```python
from build123d import *

# Parameters (mm, degrees)
SKETCH2_R               = 14.3129
SKETCH2_R_2             = 3.175
SKETCH2_R_3             = 2.6035
SKETCH2_R_4             = 3.2639
BOSS_EXTRUDE1_DEPTH     = 9.525
CHAMFER1_SIZE           = 4.7625
SKETCH3_R               = 2.6035
CUT_EXTRUDE1_DEPTH      = 25.4
CUT_EXTRUDE2_REACH      = 290.278
CUT_EXTRUDE2_END_RADIUS = 14.3129
SKETCH4_R               = 2.6035


with BuildPart() as part:
    # Sketch2 → Boss-Extrude1 (new body)
    with BuildSketch(Plane(origin=(-47.625, 0, 0), x_dir=(0, 0, -1), z_dir=(1, 0, 0))):
        with BuildLine():
            Line((51.301650802, 73.15), (51.301650802, 85.85))
            Line((51.301650802, 85.85), (24.65662816, 193.550056376))
            ThreePointArc((24.65662816, 193.550056376), (0, 212.85), (-24.65662816, 193.550056376))
            Line((-24.65662816, 193.550056376), (-51.301650802, 85.85))
            Line((-51.301650802, 85.85), (-51.301650802, 73.15))
            Line((-51.301650802, 73.15), (-51.301650802, -66.8))
            Line((-51.301650802, -66.8), (51.301650802, -66.8))
            Line((51.301650802, -66.8), (51.301650802, 73.15))
        make_face()
        with Locations(Location((0, 187.45, 0), (0, 0, 180))):
            Circle(SKETCH2_R, mode=Mode.SUBTRACT)
        with Locations(Location((38.476238101, 74.7375, 0), (0, 0, 180))):
            Circle(SKETCH2_R_2, mode=Mode.SUBTRACT)
        with Locations(Location((0, 74.7375, 0), (0, 0, 180))):
            Circle(SKETCH2_R_2, mode=Mode.SUBTRACT)
        with Locations(Location((-38.476238101, 74.7375, 0), (0, 0, 180))):
            Circle(SKETCH2_R_2, mode=Mode.SUBTRACT)
        with Locations(Location((0, 136.65, 0), (0, 0, 180))):
            Circle(SKETCH2_R_3, mode=Mode.SUBTRACT)
        with Locations(Location((-25.4, 136.65, 0), (0, 0, 180))):
            Circle(SKETCH2_R_3, mode=Mode.SUBTRACT)
        with Locations(Location((-31.75, 104.9, 0), (0, 0, 180))):
            Circle(SKETCH2_R_3, mode=Mode.SUBTRACT)
        with Locations(Location((0, 104.9, 0), (0, 0, 180))):
            Circle(SKETCH2_R_3, mode=Mode.SUBTRACT)
        with Locations(Location((31.75, 104.9, 0), (0, 0, 180))):
            Circle(SKETCH2_R_3, mode=Mode.SUBTRACT)
        with Locations(Location((25.4, 136.65, 0), (0, 0, 180))):
            Circle(SKETCH2_R_3, mode=Mode.SUBTRACT)
        with Locations(Location((-25.4, 155.7, 0), (0, 0, 180))):
            Circle(SKETCH2_R_4, mode=Mode.SUBTRACT)
        with Locations(Location((25.4, 155.7, 0), (0, 0, 180))):
            Circle(SKETCH2_R_4, mode=Mode.SUBTRACT)
    extrude(amount=BOSS_EXTRUDE1_DEPTH)

    # Chamfer1
    chamfer1_edges = [part.edges().sort_by_distance(p)[0] for p in [
        (-47.625, 74.7375, -3.175),
        (-47.625, 74.7375, -41.651238101),
        (-47.625, 74.7375, 35.301238101),
    ]]
    chamfer(chamfer1_edges, length=CHAMFER1_SIZE)

    # Sketch3 → Cut-Extrude1 (cut)
    with BuildSketch(Plane.XZ.offset(66.8)):
        with Locations(Location((-42.8625, -38.476238101, 0), (0, 0, 270))):
            Circle(SKETCH3_R)
        with Locations(Location((-42.8625, 0, 0), (0, 0, 270))):
            Circle(SKETCH3_R)
        with Locations(Location((-42.8625, 38.476238101, 0), (0, 0, 90))):
            Circle(SKETCH3_R)
    extrude(amount=-CUT_EXTRUDE1_DEPTH, mode=Mode.SUBTRACT)

    # Cut-Extrude2: up to this cylinder (the profile starts outside it)
    cut_extrude2_end = Plane(origin=(-42.8625, 187.45, 0), z_dir=(-1, 0, 0)) * Cylinder(CUT_EXTRUDE2_END_RADIUS, 610.1818, mode=Mode.PRIVATE)
    # Sketch4 → Cut-Extrude2 (cut, up to the surface)
    with BuildSketch(Plane(origin=(0, 212.85, 0), x_dir=(-1, 0, 0), z_dir=(0, 1, 0)), mode=Mode.PRIVATE) as cut_extrude2_sk1:
        with Locations(Location((42.8625, 0, 0), (0, 0, 270))):
            Circle(SKETCH4_R)
    cut_extrude2_tool1 = extrude(cut_extrude2_sk1.sketch, amount=-CUT_EXTRUDE2_REACH, mode=Mode.PRIVATE) - cut_extrude2_end
    add(cut_extrude2_tool1.solids().sort_by_distance((-42.8625, 212.85, 0))[0], mode=Mode.SUBTRACT)


solid = part.part
```
CAD build for the part. Positions are in the model's coordinates, mm. A direction names the side the tool comes from. Round coordinates to 2 decimals unless told otherwise and drop trailing zeros. Write each loop counter-clockwise with the first axis right and the second up, starting at its lowest first coordinate (ties: lowest second). Pieces come first, ordered by that corner, then holes. Notation, with made-up numbers: (-9.75, 52) - (23.25, 52) arc R8 ccw to (23.25, 56) - close; hole circle Ø10 at (-22.75, -14). An arc over 180 degrees is marked (long way). Return JSON: item names as keys, results as strings. Group by question number.
Item 1: Band-saw the part on A-A on y = 136.65. List the corners of the cut face in (x, z) (1 decimal), plus the area to 3 significant figures.
Item 2: 3-axis set-ups, long thin cutter, end or side, ignore diameter. For faces 1 (the face through (-45.172, -54.278, -1.201)), 2 (the face through (-38.1, 44, 1)): which of +Z, -Z, +X, -X, +Y, -Y reach the whole face in a straight line?
Item 3: Probe probe 1 along Y at (x, z) = (-41.4, 0); probe 2 along Z at (x, y) = (-42, -45); probe 3 along Z at (x, y) = (-44.25, -42.5). List the from-to ranges inside material, lowest first.
Item 4: Band-saw the part on B-B on z = 0. State how many separate pieces and enclosed holes the cut face has, plus the area to 3 significant figures.
Item 5: Mould opens along X. For faces 3 (the face through (-42.93, 134.07, -0.34)), 4 (the face through (-40.32, 207.27, 0.56)), 5 (the face through (-43.16, 76.85, 35.72)) say: +X half, -X half, draft (parallel to the pull), parting line (faces both ways), or undercut.
Item 6: Flat gauge pins, fed straight in: pin 1 Ø1.6 at (x, z) = (-41.5, -1) entering from -Y; pin 2 Ø1.5 at (x, z) = (-39, -21) entering from +Y; pin 3 Ø10 at (y, z) = (74.74, 0) entering from -X. Where does each tip first touch, or does it go through?
Resolved:
{
 "1": {"outline": "(-47.6, -38.7) - (-38.1, -38.7) - (-38.1, -28) - (-47.6, -28) - close; (-47.6, -22.8) - (-38.1, -22.8) - (-38.1, -2.6) - (-47.6, -2.6) - close; (-47.6, 2.6) - (-38.1, 2.6) - (-38.1, 22.8) - (-47.6, 22.8) - close; (-47.6, 28) - (-38.1, 28) - (-38.1, 38.7) - (-47.6, 38.7) - close", "area": "589 mm²"},
 "2": {"face 1": "-Y", "face 2": "+Z, -Z, +X, +Y, -Y"},
 "3": {"probe 1": "y = -41.4 to 71.56, 77.91 to 102.3, 107.5 to 134.05, 139.25 to 173.14", "probe 2": "z = -51.3 to -40.93, -36.02 to -2.46, 2.46 to 36.02, 40.93 to 51.3", "probe 3": "z = -51.3 to -40.68, -36.27 to -2.2, 2.2 to 36.27, 40.68 to 51.3"},
 "4": {"separate pieces": "6", "enclosed holes": "0", "area": "2,020 mm²"},
 "5": {"face 3": "draft", "face 4": "undercut", "face 5": "-X half"},
 "6": {"pin 1": "stops at y = -41.4", "pin 2": "stops at y = 202.78", "pin 3": "stops at x = -44.69"}
}
